For this review, take the finished solid that the model builds, in its own axes (mm). A direction names the side the tool comes from. Give positions to 0.01 mm unless a question says otherwise; leave off trailing zeros. Loops run counter-clockwise (first coordinate to the right, second up) from the corner with the lowest first, then second, coordinate; pieces in that order, holes last. Notation, with made-up numbers: (14.25, 47.25) -> (35.25, 47.25) arc R20 ccw to (35.25, 68.25) -> close; hole circle Ø5 at (-3.5, 83). An arc over 180 degrees is marked (long way). Answer as CSV lines item,"result". Start each with the question number.
Item 1: Add section B-B on z = 8. State the section outline as (x, y) points, plus the area to 3 significant figures.
Item 2: Add section C-C on y = 10. State the section outline as (x, z) points, plus the area to 3 significant figures.
Item 3: Machinability: for faces 1 (the face through (46.57, 21.15, 6.18)), 2 (the face through (-44.4, -19.08, 6.06)), which of the approach directions +Z, -Z, +X, -X, +Y, -Y give a long, thin tool a straight path to every point of the face, cutting with its end or side? Answer none if there is none.
Item 4: Clearance check with a flat-ended pin moving along its axis: P1, Ø12, axis at x = -15.5, y = -4, coming from the +Z side. State where the tip first meets the part, or that it passes through.
Item 5: Add section A-A on x = 1. State the section outline as (y, z) points.
Item 6: The part is to be moulded in two halves that separate along X. For faces 3 (the face through (-1, -6, 0)), 4 (the face through (48, -4, 5)), 5 (the face through (45, 0, 6)), 6 (the face through (-1, 0, 2)), say which applies: +X half, -X half, draft (parallel to the pull), parting line (faces both ways), or undercut.
Item 7: For L1, parallel to X at y = 1, z = 5.75; L2, parallel to Y at x = 24, z = 6.75; L3, parallel to Z at x = -31, y = 2, list the stretches that pass through material, from the lowest coordinate up. Write a range as from..to.
Item 8: Add section D-D on z = 3.5. State the section outline as (x, y) points.
```python
from build123d import *

# Parameters (mm, degrees)
F0_W     = 90
F0_H     = 39.3
F1_DEPTH = 10
F2_DEPTH = 2
F3_R     = 5
F4_R     = 2


with BuildPart() as f1:
    # F0 (on Top) → F1 (new body)
    with BuildSketch(Plane.XY):
        Polygon((-45, -29.65), (45, -29.65), (48, -29.65), (48, 19.65), (48, 22.65), (-48, 22.65), (-48, 19.65), (-48, -29.65), align=None)
        Rectangle(F0_W, F0_H, mode=Mode.SUBTRACT)
    extrude(amount=F1_DEPTH)

    # F0 (on Top) → F2 (join)
    with BuildSketch(Plane.XY):
        Rectangle(F0_W, F0_H)
    extrude(amount=F2_DEPTH)

    # F3
    f3_edges = [f1.edges().sort_by_distance(p)[0] for p in [
        (0, 22.65, 0),
        (-48, 22.65, 5),
        (48, 22.65, 5),
        (-48, -29.65, 5),
        (48, -29.65, 5),
    ]]
    fillet(f3_edges, radius=F3_R)

    # F4
    f4_edges = [f1.edges().sort_by_distance(p)[0] for p in [
        (-45, 19.65, 6),
        (45, 19.65, 6),
        (45, -19.65, 6),
        (-45, -19.65, 6),
    ]]
    fillet(f4_edges, radius=F4_R)


solid = f1.part
```
Computed values:
1,outline,"(-48, -24.65) arc R5 ccw to (-43, -29.65) -> (43, -29.65) arc R5 ccw to (48, -24.65) -> (48, 17.65) arc R5 ccw to (43, 22.65) -> (-43, 22.65) arc R5 ccw to (-48, 17.65) -> close; hole (-45, -17.65) arc R2 ccw to (-43, -19.65) -> (43, -19.65) arc R2 ccw to (45, -17.65) -> (45, 17.65) arc R2 ccw to (43, 19.65) -> (-43, 19.65) arc R2 ccw to (-45, 17.65) -> close"
1,area,"1,470 mm²"
2,outline,"(-48, 0) -> (48, 0) -> (48, 10) -> (45, 10) -> (45, 2) -> (-45, 2) -> (-45, 10) -> (-48, 10) -> close"
2,area,"240 mm²"
3,face 1,"+Z, -Z, +X, +Y"
3,face 2,"+Z"
4,P1,"z = 2"
5,outline,"(-29.65, 0) -> (17.65, 0) arc R5 ccw to (22.65, 5) -> (22.65, 10) -> (19.65, 10) -> (19.65, 2) -> (-19.65, 2) -> (-19.65, 10) -> (-29.65, 10) -> close"
6,face 3,"draft"
6,face 4,"+X half"
6,face 5,"undercut"
6,face 6,"undercut"
7,L1,"-48..-45, 45..48"
7,L2,"-29.65..-19.65, 19.65..22.65"
7,L3,"0..2"
8,outline,"(-48, -24.65) arc R5 ccw to (-43, -29.65) -> (43, -29.65) arc R5 ccw to (48, -24.65) -> (48, 17.65) arc R5 ccw to (44.5, 22.42) -> (-44.5, 22.42) arc R5 ccw to (-48, 17.65) -> close; hole (-45, -17.65) arc R2 ccw to (-43, -19.65) -> (43, -19.65) arc R2 ccw to (45, -17.65) -> (45, 17.65) arc R2 ccw to (43, 19.65) -> (-43, 19.65) arc R2 ccw to (-45, 17.65) -> close"
